```python
from build123d import *

# Parameters (mm, degrees)
BOX069_W          = 4
BOX069_H          = 3.5
BOX069_DEPTH      = 4
BOX065_W          = 7
BOX065_H          = 6.5
BOX065_DEPTH      = 3
CHAMFER_SIZE      = 0.99
BOX074_W          = 7
BOX074_H          = 6
BOX074_DEPTH      = 3
SKETCH001_W       = 30
SKETCH001_H       = 40
SKETCH001_W_2     = 28
SKETCH001_H_2     = 38
PAD001_DEPTH      = 2
CYLINDER015_R     = 2.8
CYLINDER015_DEPTH = 3
CYLINDER014_R     = 2.8
CYLINDER014_DEPTH = 3
CYLINDER013_R     = 2.8
CYLINDER013_DEPTH = 3
CYLINDER016_R     = 2.8
CYLINDER016_DEPTH = 3
BOX014_W          = 4
BOX014_H          = 3.5
BOX014_DEPTH      = 4
BOX015_W          = 4
BOX015_H          = 3.5
BOX015_DEPTH      = 4
CYLINDER010_R     = 1.8
CYLINDER010_DEPTH = 6
CYLINDER011_R     = 1.8
CYLINDER011_DEPTH = 6
CYLINDER012_R     = 1.8
CYLINDER012_DEPTH = 6
CYLINDER009_R     = 1.8
CYLINDER009_DEPTH = 6
BOX042_W          = 44
BOX042_H          = 44
BOX042_DEPTH      = 4


with BuildPart() as button2_box0002:
    # Box069 → Box069 (new body)
    with BuildSketch(Plane(origin=(13, 19, 19), x_dir=(1, 0, 0), z_dir=(0, 0, 1))):
        with Locations((2, 1.75)):
            Rectangle(BOX069_W, BOX069_H)
    extrude(amount=BOX069_DEPTH)


with BuildPart() as cut006:
    # Box065 → Box065 (new body)
    with BuildSketch(Plane(origin=(11.5, 17.5, 21), x_dir=(1, 0, 0), z_dir=(0, 0, 1))):
        with Locations((3.5, 3.25)):
            Rectangle(BOX065_W, BOX065_H)
    extrude(amount=BOX065_DEPTH)

    # Chamfer
    chamfer_edges = [cut006.edges().sort_by_distance(p)[0] for p in [
        (11.5, 20.75, 24),
        (18.5, 20.75, 24),
        (15, 17.5, 24),
        (15, 24, 24),
    ]]
    chamfer(chamfer_edges, length=CHAMFER_SIZE)

    # Cut006: cut Button2_box0002
    add(button2_box0002.part, mode=Mode.SUBTRACT)


with BuildPart() as cone001:
    # Cone001 → Cone001 (revolve)
    with BuildSketch(Plane(origin=(15, 9.75, 21), x_dir=(1, 0, 0), z_dir=(0, -1, 0))):
        Polygon((0, 0), (2.4, 0), (1.5, 1), (0, 1), align=None)
    revolve(axis=Axis((15, 9.75, 21), (0, 0, 1)))


with BuildPart() as button_top_cover001:
    # Cone → Cone (revolve)
    with BuildSketch(Plane(origin=(15, 9.75, 21), x_dir=(1, 0, 0), z_dir=(0, -1, 0))):
        Polygon((0, 0), (3, 0), (1.7, 1.3), (0, 1.3), align=None)
    revolve(axis=Axis((15, 9.75, 21), (0, 0, 1)))

    # Cut003: cut Cone001
    add(cone001.part, mode=Mode.SUBTRACT)


with BuildPart() as button_top_cover001_1:
    # Cut003 placement: moved
    add(button_top_cover001.part.moved(Location((0, 0, 2))))


with BuildPart() as box074:
    # Box074 → Box074 (new body)
    with BuildSketch(Plane(origin=(11.5, 28.75, 20.6), x_dir=(1, 0, 0), z_dir=(0, 0, 1))):
        with Locations((3.5, 3)):
            Rectangle(BOX074_W, BOX074_H)
    extrude(amount=BOX074_DEPTH)


with BuildPart() as gasket_cut:
    # Sketch001 → Pad001 (new body)
    with BuildSketch(Plane(origin=(2, 2, 19), x_dir=(1, 0, 0), z_dir=(0, 0, 1))):
        with Locations((13, 18)):
            Rectangle(SKETCH001_W, SKETCH001_H)
        with Locations((13, 18)):
            Rectangle(SKETCH001_W_2, SKETCH001_H_2, mode=Mode.SUBTRACT)
    extrude(amount=PAD001_DEPTH)


with BuildPart() as screw_head003:
    # Cylinder015 → Cylinder015 (new body)
    with BuildSketch(Plane(origin=(33, 38, 21), x_dir=(1, 0, 0), z_dir=(0, 0, 1))):
        Circle(CYLINDER015_R)
    extrude(amount=CYLINDER015_DEPTH)


with BuildPart() as screw_head002:
    # Cylinder014 → Cylinder014 (new body)
    with BuildSketch(Plane(origin=(-3, 38, 21), x_dir=(1, 0, 0), z_dir=(0, 0, 1))):
        Circle(CYLINDER014_R)
    extrude(amount=CYLINDER014_DEPTH)


with BuildPart() as screw_head001:
    # Cylinder013 → Cylinder013 (new body)
    with BuildSketch(Plane(origin=(-3, 2, 21), x_dir=(1, 0, 0), z_dir=(0, 0, 1))):
        Circle(CYLINDER013_R)
    extrude(amount=CYLINDER013_DEPTH)


with BuildPart() as screw_head_cut:
    # Cylinder016 → Cylinder016 (new body)
    with BuildSketch(Plane(origin=(33, 2, 21), x_dir=(1, 0, 0), z_dir=(0, 0, 1))):
        Circle(CYLINDER016_R)
    extrude(amount=CYLINDER016_DEPTH)

    # Fusion019: union Screw_head003, Screw_head002, Screw_head001
    add(screw_head003.part)
    add(screw_head002.part)
    add(screw_head001.part)


with BuildPart() as button1_box0001:
    # Box014 → Box014 (new body)
    with BuildSketch(Plane(origin=(13, 8, 19), x_dir=(1, 0, 0), z_dir=(0, 0, 1))):
        with Locations((2, 1.75)):
            Rectangle(BOX014_W, BOX014_H)
    extrude(amount=BOX014_DEPTH)


with BuildPart() as fusion004_cut:
    # Box015 → Box015 (new body)
    with BuildSketch(Plane(origin=(13, 19, 19), x_dir=(1, 0, 0), z_dir=(0, 0, 1))):
        with Locations((2, 1.75)):
            Rectangle(BOX015_W, BOX015_H)
    extrude(amount=BOX015_DEPTH)

    # Fusion004: union Button1_box0001
    add(button1_box0001.part)


with BuildPart() as obj1:
    # Cylinder010 → Cylinder010 (new body)
    with BuildSketch(Plane(origin=(-3, 38, 15), x_dir=(1, 0, 0), z_dir=(0, 0, 1))):
        Circle(CYLINDER010_R)
    extrude(amount=CYLINDER010_DEPTH)


with BuildPart() as obj2:
    # Cylinder011 → Cylinder011 (new body)
    with BuildSketch(Plane(origin=(33, 2, 15), x_dir=(1, 0, 0), z_dir=(0, 0, 1))):
        Circle(CYLINDER011_R)
    extrude(amount=CYLINDER011_DEPTH)


with BuildPart() as obj3:
    # Cylinder012 → Cylinder012 (new body)
    with BuildSketch(Plane(origin=(33, 38, 15), x_dir=(1, 0, 0), z_dir=(0, 0, 1))):
        Circle(CYLINDER012_R)
    extrude(amount=CYLINDER012_DEPTH)


with BuildPart() as top_cut:
    # Cylinder009 → Cylinder009 (new body)
    with BuildSketch(Plane(origin=(-3, 2, 15), x_dir=(1, 0, 0), z_dir=(0, 0, 1))):
        Circle(CYLINDER009_R)
    extrude(amount=CYLINDER009_DEPTH)

    # Fusion018: union obj1, obj2, obj3
    add(obj1.part)
    add(obj2.part)
    add(obj3.part)

    # Fusion020: union Gasket_cut, Screw_Head_cut, Fusion004_cut
    add(gasket_cut.part)
    add(screw_head_cut.part)
    add(fusion004_cut.part)


with BuildPart() as top_final:
    # Box042 → Box042 (new body)
    with BuildSketch(Plane(origin=(-7, -2, 19), x_dir=(1, 0, 0), z_dir=(0, 0, 1))):
        with Locations((22, 22)):
            Rectangle(BOX042_W, BOX042_H)
    extrude(amount=BOX042_DEPTH)

    # Cut004: cut top_cut
    add(top_cut.part, mode=Mode.SUBTRACT)

    # Cut010: cut Box074
    add(box074.part, mode=Mode.SUBTRACT)

    # Fusion025: union Cut006, Button_Top_cover001
    add(cut006.part)
    add(button_top_cover001_1.part)


solid = top_final.part
```
Source: CAD feature listing. Evaluate the final solid. Frame: model axes, mm. A direction names the side the tool comes from. Give positions to 0.01 mm unless a question says otherwise; leave off trailing zeros. Order: outer loops, then holes, each group sorted by start corner. A loop starts at its lowest first (then second) coordinate and runs counter-clockwise, first axis right, second up.
(1) Contact query for flat-ended pins moving along their axis: P1, Ø3, axis at x = -4, y = 2, coming from the +Z side; P2, Ø6, axis at x = 32, y = 37.5, coming from the +Z side. Output: stop coordinate, or through.
(2) Section query D-D (x = 0.5). Return the cut outline in (y, z).
(3) Section query A-A (x = 33). Return the cut outline in (y, z).
(4) Pull-direction query (Y, two-part tool) for faces 1 (the face through (29, 20, 20)), 2 (the face through (37, 20, 21)), 3 (the face through (15, -2, 21)); classes: +Y half, -Y half, draft (parallel to the pull), parting line (faces both ways), or undercut.
(5) Section query C-C (z = 19.75). State how many separate pieces and enclosed holes the cut face has, plus the area to 3 significant figures.
(6) Access query for faces 4 (the face through (15, 32, 20.6)), 5 (the face through (15, 21, 24)), 6 (the face through (15, 21, 23)). Directions: +Z, -Z, +X, -X, +Y, -Y. A direction counts if a zero-diameter tool reaches every point of the face in a straight line with its end or side. Return the directions, or none.
(7) Section query B-B (y = 2). Return the cut outline in (x, z).
(8) Material intervals for line 1 along Y through (x, z) = (33, 20.4); line 2 along Y through (x, z) = (-3, 21.8); line 3 along X through (y, z) = (9, 20.05), sorted ascending.
Outcome:
1. P1: stops at z = 21
1. P2: stops at z = 23
2. outline: (-2, 19) - (0, 19) - (0, 21) - (40, 21) - (40, 19) - (42, 19) - (42, 23) - (-2, 23) - close
3. outline: (-2, 19) - (0.2, 19) - (0.2, 21) - (-0.8, 21) - (-0.8, 23) - (-2, 23) - close; (3.8, 19) - (36.2, 19) - (36.2, 21) - (35.2, 21) - (35.2, 23) - (4.8, 23) - (4.8, 21) - (3.8, 21) - close; (39.8, 19) - (42, 19) - (42, 23) - (40.8, 23) - (40.8, 21) - (39.8, 21) - close
4. face 1: undercut
4. face 2: draft
4. face 3: -Y half
5. separate pieces: 2
5. enclosed holes: 7
5. area: 1,730 mm2
6. face 4: +Z
6. face 5: +Z, +X, -X, +Y
6. face 6: -Z
7. outline: (-7, 19) - (-4.8, 19) - (-4.8, 21) - (-5.8, 21) - (-5.8, 23) - (-7, 23) - close; (-1.2, 19) - (0, 19) - (0, 21) - (1, 21) - (1, 19) - (29, 19) - (29, 21) - (30, 21) - (30, 19) - (31.2, 19) - (31.2, 21) - (30.2, 21) - (30.2, 23) - (-0.2, 23) - (-0.2, 21) - (-1.2, 21) - close; (34.8, 19) - (37, 19) - (37, 23) - (35.8, 23) - (35.8, 21) - (34.8, 21) - close
8. line 1: y = -2 to 0.2, 3.8 to 36.2, 39.8 to 42
8. line 2: y = -2 to -0.8, 4.8 to 35.2, 40.8 to 42
8. line 3: x = -7 to 0, 1 to 13, 17 to 29, 30 to 37
